Build history of the part. All positions in model axes, mm. A direction names the side the tool comes from. Round coordinates to 2 decimals unless told otherwise and drop trailing zeros. Loops run counter-clockwise (first coordinate to the right, second up) from the corner with the lowest first, then second, coordinate; pieces in that order, holes last. Notation, with made-up numbers: M 63.5,-38 L 121.5,-38 A18 ccw 121.5,-29 Z; hole C 33.5,-16 d10. An arc over 180 degrees is marked long. One line per item, written item: value.
Autodesk Fusion 360 part; units mm, degrees
sketch "3D-printed conduit outline" plane through (0, 0, 0) normal (0, 1, 0) x (1, 0, 0)
  line L0 (0, 0) -> (16, 0)
  line L1 (16, 0) -> (16, -14)
  line L2 (16, -14) -> (0, -14)
  line L3 (0, -14) -> (0, 0)
  line L4 (2, -14) -> (14, -14)
  line L5 (14, -14) -> (14, -2)
  line L6 (14, -2) -> (2, -2)
  line L7 (2, -2) -> (2, -14)
  dimension "d8" = 14
  dimension "d9" = 16
  dimension "d10" = 2
  dimension "d11" = 2
  dimension "d12" = 2
extrude "Extrude1" add sketch "3D-printed conduit outline" along normal blind 201 contours L0 L1 L2 L3 L5 L6 L7
sketch "Magnet holders" plane through (0, 0, 14) normal (0, 0, 1) x (-1, 0, 0)
  line L0 (0, 0) -> (-2, 0)
  line L1 (-2, 0) -> (-2, -201)
  line L2 (-2, -201) -> (0, -201)
  line L3 (0, -201) -> (0, 0)
  line L4 (-14, 0) -> (-16, 0)
  line L5 (-16, 0) -> (-16, -201)
  line L6 (-16, -201) -> (-14, -201)
  line L7 (-14, -201) -> (-14, 0)
  circle A0 centre (-2.5, -2.5) radius 2.5
  circle A1 centre (-2.5, -2.5) radius 1.75
  line L8 (-14, 0) -> (-2, 0)
  line L9 (0, 0) -> (-2.5, 0)
  line L10 (-2.5, 0) -> (-2.5, -5)
  line L11 (-2.5, -5) -> (0, -5)
  line L12 (0, -5) -> (0, 0)
  circle A2 centre (-13.5, -2.5) radius 2.5
  circle A3 centre (-13.5, -2.5) radius 1.75
  line L13 (-16, 0) -> (-13.5, 0)
  line L14 (-13.5, 0) -> (-13.5, -5)
  line L15 (-13.5, -5) -> (-16, -5)
  line L16 (-16, -5) -> (-16, 0)
  circle A4 centre (-2.5, -63.1667) radius 1.75
  circle A5 centre (-2.5, -63.1667) radius 2.5
  line L17 (-2.5, -60.6667) -> (-2.5, -65.6667)
  line L18 (-2.5, -65.6667) -> (0, -65.6667)
  line L19 (0, -65.6667) -> (0, -60.6667)
  line L20 (0, -60.6667) -> (-2.5, -60.6667)
  circle A6 centre (-13.5, -63.1667) radius 1.75
  circle A7 centre (-13.5, -63.1667) radius 2.5
  line L21 (-13.5, -60.6667) -> (-13.5, -65.6667)
  line L22 (-13.5, -65.6667) -> (-16, -65.6667)
  line L23 (-16, -65.6667) -> (-16, -60.6667)
  line L24 (-16, -60.6667) -> (-13.5, -60.6667)
  circle A8 centre (-2.5, -123.8333) radius 1.75
  circle A9 centre (-2.5, -123.8333) radius 2.5
  line L25 (-2.5, -121.3333) -> (-2.5, -126.3333)
  line L26 (-2.5, -126.3333) -> (0, -126.3333)
  line L27 (0, -126.3333) -> (0, -121.3333)
  line L28 (0, -121.3333) -> (-2.5, -121.3333)
  circle A10 centre (-13.5, -123.8333) radius 1.75
  circle A11 centre (-13.5, -123.8333) radius 2.5
  line L29 (-13.5, -121.3333) -> (-13.5, -126.3333)
  line L30 (-13.5, -126.3333) -> (-16, -126.3333)
  line L31 (-16, -126.3333) -> (-16, -121.3333)
  line L32 (-16, -121.3333) -> (-13.5, -121.3333)
  circle A12 centre (-2.5, -184.5) radius 1.75
  circle A13 centre (-2.5, -184.5) radius 2.5
  line L33 (-2.5, -182) -> (-2.5, -187)
  line L34 (-2.5, -187) -> (0, -187)
  line L35 (0, -187) -> (0, -182)
  line L36 (0, -182) -> (-2.5, -182)
  circle A14 centre (-13.5, -184.5) radius 1.75
  circle A15 centre (-13.5, -184.5) radius 2.5
  line L37 (-13.5, -182) -> (-13.5, -187)
  line L38 (-13.5, -187) -> (-16, -187)
  line L39 (-16, -187) -> (-16, -182)
  line L40 (-16, -182) -> (-13.5, -182)
  dimension "d15" = 5
  dimension "d16" = 3.5
  dimension "d17" = 5
  dimension "d18" = 3.5
  dimension "d21" = 0
  dimension "d22" = -182
sketch "End wall" plane through (0, 201, 0) normal (0, 1, 0) x (-1, 0, 0)
  line L0 (-2, 2) -> (-14, 2)
  line L1 (-14, 2) -> (-14, 14)
  line L2 (-14, 14) -> (-16, 14)
  line L3 (-16, 14) -> (-16, 0)
  line L4 (-16, 0) -> (0, 0)
  line L5 (0, 0) -> (0, 14)
  line L6 (0, 14) -> (-2, 14)
  line L7 (-2, 14) -> (-2, 2)
  line L8 (-16, 0) -> (0, 0)
  line L9 (0, 0) -> (0, 14)
  line L10 (0, 14) -> (-16, 14)
  line L11 (-16, 14) -> (-16, 0)
extrude "Extrude5" add sketch "End wall" against normal blind 2
extrude "Extrude2" add sketch "Magnet holders" against normal blind 3 contours A2 A3 L14 | L7 A2 A3 L14 | L7 L8 A2 L13 | L1 A0 L8 L9 | L1 A0 A1 L10 | A0 A1 L10 | L1 A0 A1 L10 | L1 A0 L11 | L1 A1 L10 | A1 L10 | L7 A3 L14 | A3 L14 | L1 A5 L20 | L7 A2 L15 | L7 A2 A3 L14 | L1 A4 A5 L17 | L1 A4 A5 L17 | L1 A5 L18 | A4 A5 L17 | L1 A4 L17 | A4 L17 | L7 A7 L24 | L1 A9 L28 | L7 A6 A7 L21 | A6 A7 L21 | L1 A8 A9 L25 | L1 A8 A9 L25 | L1 A9 L26 | A8 A9 L25 | L7 A6 L21 | A6 L21 | L7 A7 L22 | L7 A6 A7 L21 | L1 A8 L25 | A8 L25 | L1 A13 L36 | L7 A11 L32 | L1 A12 A13 L33 | L1 A12 A13 L33 | L1 A13 L34 | A12 A13 L33 | L7 A10 A11 L29 | L7 A11 L30 | L7 A10 A11 L29 | A10 A11 L29 | L1 A12 L33 | A12 L33 | L7 A10 L29 | A10 L29 | L7 A15 L40 | L7 A14 A15 L37 | L7 A15 L38 | L7 A14 A15 L37 | A14 A15 L37 | L7 A14 L37 | A14 L37
extrude "Extrude6" cut sketch "Magnet holders" against normal blind 1 contours L1 A1 | L1 A1 L10 | A1 L10 | L7 A3 L14 | A3 L14 | L7 A3 | L1 A4 | L1 A4 L17 | A4 L17 | L7 A6 L21 | L7 A6 | A6 L21 | L1 A8 | L1 A8 L25 | A8 L25 | L1 A12 | L1 A12 L33 | A12 L33 | L7 A10 L29 | L7 A10 | A10 L29 | L7 A14 L37 | L7 A14 | A14 L37
chamfer "Chamfer2" distance 2.9999 angle 45 11 edges at (2, 2.5, 11) (2, 63.1667, 11) (2, 123.8333, 11) (2, 2.5, 11) (2, 123.8333, 11) (2, 63.1667, 11) (2, 184.5, 11) (14, 2.5, 11) (14, 63.1667, 11) (14, 123.8333, 11) (14, 184.5, 11)
sketch "Arcade button outlets" plane through (0, 0, 0) normal (-1, 0, 0) x (0, -1, 0)
  line L0 (0, 0) -> (0, 14)
  line L1 (0, 14) -> (-201, 14)
  line L2 (-201, 14) -> (-201, 0)
  line L3 (-201, 0) -> (0, 0)
  line L4 (-199, 14) -> (-187, 14)
  line L5 (-187, 14) -> (-187, 2)
  line L6 (-187, 2) -> (-199, 2)
  line L7 (-199, 2) -> (-199, 14)
  line L8 (-149, 14) -> (-137, 14)
  line L9 (-137, 14) -> (-137, 2)
  line L10 (-137, 2) -> (-149, 2)
  line L11 (-149, 2) -> (-149, 14)
  line L12 (-99, 14) -> (-87, 14)
  line L13 (-87, 14) -> (-87, 2)
  line L14 (-87, 2) -> (-99, 2)
  line L15 (-99, 2) -> (-99, 14)
  dimension "d29" = 2
  dimension "d30" = 12
  dimension "d31" = 12
  dimension "d32" = 12
  dimension "d33" = 2
  dimension "d34" = 38
  dimension "d35" = 38
extrude "Extrude4" cut sketch "Arcade button outlets" against normal blind 2 contours L1 L12 L13 L14 L15 | L1 L4 L5 L6 L7 | L1 L8 L9 L10 L11
sketch "End chamfer" plane through (0, 0, 14) normal (0, 0, 1) x (-1, 0, 0)
  line L0 (0, -199) -> (-14, -199)
  line L1 (-14, -199) -> (-14, -187)
  line L2 (-14, -187) -> (-13.5, -187)
  arc A0 (-13.5, -187) -> (-13.5, -182) centre (-13.5, -184.5) ccw
  line L3 (-13.5, -182) -> (-14, -182)
  line L4 (-14, -182) -> (-14, -126.3333)
  line L5 (-14, -126.3333) -> (-13.5, -126.3333)
  arc A1 (-13.5, -126.3333) -> (-13.5, -121.3333) centre (-13.5, -123.8333) ccw
  line L6 (-13.5, -121.3333) -> (-14, -121.3333)
  line L7 (-14, -121.3333) -> (-14, -65.6667)
  line L8 (-14, -65.6667) -> (-13.5, -65.6667)
  arc A2 (-13.5, -65.6667) -> (-13.5, -60.6667) centre (-13.5, -63.1667) ccw
  line L9 (-13.5, -60.6667) -> (-14, -60.6667)
  line L10 (-14, -60.6667) -> (-14, -5)
  line L11 (-14, -5) -> (-13.5, -5)
  arc A3 (-13.5, -5) -> (-13.5, 0) centre (-13.5, -2.5) ccw
  line L12 (-13.5, 0) -> (-16, 0)
  line L13 (-16, 0) -> (-16, -201)
  line L14 (-16, -201) -> (0, -201)
  line L15 (0, -201) -> (0, -199)
  circle A4 centre (-13.5, -2.5) radius 1.75
  circle A5 centre (-13.5, -63.1667) radius 1.75
  circle A6 centre (-13.5, -184.5) radius 1.75
  circle A7 centre (-13.5, -123.8333) radius 1.75
  line L16 (-6.8284, -201) -> (-16, -191.8284)
  line L17 (-4, -201) -> (-16, -189)
  line L18 (-2, -149) -> (-2, -182)
  line L19 (0, -193) -> (-8, -193)
  line L20 (0, -187) -> (0, -199)
  line L21 (-4, -193) -> (-8, -189)
  line L22 (-4, -193) -> (-0.3616, -193) construction
  line L23 (-8, -189) -> (-8, -193)
  line L24 (-10, -195) -> (-2, -187)
  line L25 (-2.5, -187) -> (0, -187)
  line L26 (-4, -201) -> (-6.8284, -201)
  line L27 (-16, -191.8284) -> (-16, -189)
  point P0 (-6, -191)
  dimension "d46" = 6
  dimension "d47" = 8
  dimension "d49" = 135
  dimension "d50" = 4
  dimension "d51" = 2
  dimension "d52" = 2
extrude "Extrude8" add sketch "End chamfer" against normal blind 12 contours L0 L14 L16 L17 L26 | L0 L1 L16 L17 | L1 L13 L16 L17 L27
extrude "Extrude7" cut sketch "End chamfer" against normal blind 14 contours L0 L1 L13 L14 L16 | L0 L1 L16
chamfer "Chamfer4" distance 1 angle 45 11 edges at (2, 43.5, 2) (1, 87, 2) (1, 99, 2) (2, 118, 2) (1, 137, 2) (1, 149, 2) (2, 168, 2) (1, 187, 2) (3, 199, 2) (10, 195, 2) (14, 95.5, 2)
equation "conduit_length = 201 mm"
equation "conduit_width = 16 mm"
equation "conduit_height = 16 mm"
equation "conduit_wall_thickness = 2 mm"
equation "magnet_diameter = 3 mm"
equation "magnet_height = 1 mm"
equation "d8 = conduit_height - conduit_wall_thickness"
equation "d9 = conduit_width"
equation "d10 = conduit_wall_thickness"
equation "d11 = conduit_wall_thickness"
equation "d12 = conduit_wall_thickness"
equation "d13 = conduit_length"
equation "d15 = magnet_diameter + 2 mm"
equation "d16 = magnet_diameter + 0.5 mm"
equation "d17 = magnet_diameter + 2 mm"
equation "d18 = magnet_diameter + 0.5 mm"
equation "d22 = -conduit_length + ( magnet_diameter + 2 mm ) + 14 mm"
equation "d23 = -( magnet_height + 2 mm )"
equation "d29 = conduit_wall_thickness"
equation "d33 = conduit_wall_thickness"
equation "d47 = conduit_wall_thickness + ( conduit_width - 2 * conduit_wall_thickness ) / 2"
equation "d50 = Linear Dimension-4"
equation "d51 = conduit_wall_thickness"
equation "d52 = conduit_wall_thickness"
equation "d55 = -( conduit_height - 2 * conduit_wall_thickness )"
Item 1: Slice it at A-A, the plane z = 5.5. Give the cut face in (x, y), and give its area (3 significant figures).
Check values:
outline: M 0,0 L 2,0 L 2,87 L 0,87 Z; M 0,99 L 2,99 L 2,137 L 0,137 Z; M 0,149 L 2,149 L 2,187 L 0,187 Z; M 0,199 L 6,199 L 14,191 L 14,0 L 16,0 L 16,191.83 L 6.83,201 L 0,201 Z
area: 746 mm2
Item 2: Pull direction Y, two halves, no side cores. Call faces 1 (the face through (8, 99, 0)), 2 (the face through (3, 124, 13)), 3 (the face through (11.35, 196.48, 7.1)): pulls with the +Y half, pulls with the -Y half, needs draft (parallel to the pull), parting line crosses it, or undercut.
Check values:
face 1: needs draft
face 2: undercut
face 3: pulls with the +Y half
Item 3: Which spindle directions (+Z, -Z, +X, -X, +Y, -Y) get a long thin tool onto all of the face, cutting with end or side? Do faces 4 (the face through (9.71, 194.6, 2.51)), 5 (the face through (3, 63, 13)). Say none if no direction does.
Check values:
face 4: +Z, -X, -Y
face 5: +Z
Item 4: Slice it at B-B, the plane y = 33.5. Give the cut face in (x, z), and give its area (3 significant figures).
Check values:
outline: M 0,0 L 16,0 L 16,14 L 14,14 L 14,3 L 13,2 L 3,2 L 2,3 L 2,14 L 0,14 Z
area: 81.0 mm2
Item 5: Wall check: line 1 along X through (y, z) = (2.5, 13.8); line 2 along X through (y, z) = (122.5, 7.75); line 3 along Z through (x, y) = (2.5, 148.5). Give the ranges that are in metal, low to high.
Check values:
line 1: x = 0 to 0.75, 4.25 to 5, 11 to 11.75, 15.25 to 16
line 2: x = 0 to 2, 14 to 16
line 3: z = 0 to 2.5
Item 6: Drop flat-ended pins along their axis: P1, Ø3, axis at x = 8.5, y = 124, coming from the +Z side; P2, Ø3, axis at x = 13.5, y = 2.5, coming from the +Z side; P3, Ø3, axis at y = 89.5, z = 8, coming from the -X side. Give the stop position or say it passes through.
Check values:
P1: stops at z = 2
P2: stops at z = 13
P3: stops at x = 14
